Could you check a few things on this model? Use its own coordinates, in mm. A direction names the side the tool comes from. Coordinates: 2 decimals unless noted, no trailing zeros. Loops run counter-clockwise (first coordinate to the right, second up) from the corner with the lowest first, then second, coordinate; pieces in that order, holes last. Notation, with made-up numbers: M -21,9 L 0,9 A13 cw 0,32 Z; hole C -4.75,44.25 d6. An arc over 180 degrees is marked long. Write each question's results on one line, items separated by ' | '.
Autodesk Inventor part; units mm, degrees
ref_plane "YZ Plane" through (0, 0, 0) normal (1, 0, 0) x (0, 1, 0)
ref_plane "XZ Plane" through (0, 0, 0) normal (0, 1, 0) x (-1, 0, 0)
ref_plane "XY Plane" through (0, 0, 0) normal (0, 0, 1) x (1, 0, 0)
ref_plane "РабПлоскость1" through (0, 0, 0) normal (0, 0, 1) x (1, 0, 0)
sketch "Эскиз1" plane through (0, 0, 0) normal (0, 0, 1) x (1, 0, 0)
  circle A0 centre (190, 44.9968) radius 4
  circle A1 centre (190, 89.9937) radius 4
  circle A2 centre (177.9182, 131.4529) radius 4
  circle A3 centre (134.9905, 140) radius 4
  circle A4 centre (89.9937, 140) radius 4
  circle A5 centre (44.9968, 140) radius 4
  circle A6 centre (0, 140) radius 4
  circle A7 centre (-44.9968, 140) radius 4
  circle A8 centre (-89.9937, 140) radius 4
  circle A9 centre (-134.9905, 140) radius 4
  circle A10 centre (-177.9182, 131.4529) radius 4
  circle A11 centre (-190, 89.9937) radius 4
  circle A12 centre (-190, 44.9968) radius 4
  circle A13 centre (-190, 0) radius 4
  circle A14 centre (-190, -44.9968) radius 4
  circle A15 centre (-190, -89.9937) radius 4
  circle A16 centre (-177.9182, -131.4529) radius 4
  circle A17 centre (-134.9905, -140) radius 4
  circle A18 centre (-89.9937, -140) radius 4
  circle A19 centre (-44.9968, -140) radius 4
  circle A20 centre (0, -140) radius 4
  circle A21 centre (44.9968, -140) radius 4
  circle A22 centre (89.9937, -140) radius 4
  circle A23 centre (134.9905, -140) radius 4
  circle A24 centre (177.9182, -131.4529) radius 4
  circle A25 centre (190, -89.9937) radius 4
  circle A26 centre (190, -44.9968) radius 4
  circle A27 centre (190, 0) radius 4
  line L0 (-200, -110) -> (-200, 110)
  arc A28 (-200, -110) -> (-160, -150) centre (-160, -110) ccw
  line L1 (160, -150) -> (-160, -150)
  arc A29 (160, -150) -> (200, -110) centre (160, -110) ccw
  line L2 (200, 110) -> (200, -110)
  arc A30 (200, 110) -> (160, 150) centre (160, 110) ccw
  line L3 (-160, 150) -> (160, 150)
  arc A31 (-160, 150) -> (-200, 110) centre (-160, 110) ccw
  line L4 (-150, -130) -> (150, -130)
  arc A32 (-180, -100) -> (-150, -130) centre (-150, -100) ccw
  line L5 (-180, 100) -> (-180, -100)
  arc A33 (-150, 130) -> (-180, 100) centre (-150, 100) ccw
  line L6 (150, 130) -> (-150, 130)
  arc A34 (180, 100) -> (150, 130) centre (150, 100) ccw
  line L7 (180, -100) -> (180, 100)
  arc A35 (150, -130) -> (180, -100) centre (150, -100) ccw
  point P0 (0, 0)
extrude "Выдавливание1" add sketch "Эскиз1" along normal blind 2
properties part number "Прокладка крышки фонаря 1" material "Алюминий 6061"
(1) Imagine slicing it at C-C, the plane z = 0.6. State how many separate pieces and enclosed holes the cut face has, and give its area (3 significant figures).
Reported:
separate pieces: 1 | enclosed holes: 29 | area: 24,400 mm2
(2) Imagine slicing it at B-B, the plane x = 167.5. List the corners of the cut face in (y, z) for me, and give its area (3 significant figures).
Reported:
outline: M -149.29,0 L -124.37,0 L -124.37,2 L -149.29,2 Z; M 124.37,0 L 149.29,0 L 149.29,2 L 124.37,2 Z | area: 99.7 mm2
(3) Please list where these lines run through material, in increasing order: probe 1 along Y at (x, z) = (67, 1.4); probe 2 along Y at (x, z) = (131.5, 0.1); probe 3 along Y at (x, z) = (190, 1.05). Write a range as from..to.
Reported:
probe 1: y = -150..-130, 130..150 | probe 2: y = -150..-141.95, -138.05..-130, 130..138.05, 141.95..150 | probe 3: y = -136.46..-93.99, -85.99..-49, -41..-4, 4..41, 49..85.99, 93.99..136.46
(4) If we mould it in two halves opening along Y, with no side actions, what happens to faces 3 (the cylindrical face through (193.695, 91.526, 0.986)), 4 (the flat face through (-1, 134, 0)), 5 (the cylindrical face through (187.972, 138.594, 0.986))? For each: released by +Y, released by -Y, zero draft, split by the parting line, or undercut.
Reported:
face 3: undercut | face 4: zero draft | face 5: released by +Y
(5) Which directions (+Z, -Z, +X, -X, +Y, -Y) give clear straight access to the entire face, cutting with the end or side of a thin tool? Please do faces 1 (the cylindrical face through (188.594, -137.972, 0.986)), 2 (the cylindrical face through (170.979, 121.445, 0.986)).
Reported:
face 1: +Z, -Z, +X, -Y | face 2: +Z, -Z
(6) Imagine slicing it at A-A, the plane x = -113. List the corners of the cut face in (y, z) for me, and give its area (3 significant figures).
Reported:
outline: M -150,0 L -130,0 L -130,2 L -150,2 Z; M 130,0 L 150,0 L 150,2 L 130,2 Z | area: 80.0 mm2
(7) Will this pin go through, and if not, where does the flat tip stop? P1, Ø5, axis at x = 190, y = -45, coming from the -Z side.
Reported:
P1: passes through
